Input: part model. Units: mm. Frame: model coordinates. A direction names the side the tool comes from. Coordinates: 2 decimals unless noted, no trailing zeros. Order: outer loops, then holes, each group sorted by start corner. A loop starts at its lowest first (then second) coordinate and runs counter-clockwise, first axis right, second up. Notation, with made-up numbers: M 52,31.5 L 68,31.5 A22 cw 68,40.5 Z; hole C 39.5,69.5 d5. An arc over 180 degrees is marked long. One line per item, written item: value.
Autodesk Inventor part; units mm, degrees
ref_plane "YZ Plane" through (0, 0, 0) normal (1, 0, 0) x (0, 1, 0)
ref_plane "XZ Plane" through (0, 0, 0) normal (0, 1, 0) x (-1, 0, 0)
ref_plane "XY Plane" through (0, 0, 0) normal (0, 0, 1) x (1, 0, 0)
sketch "Эскиз1" plane through (0, 0, 0) normal (0, 1, 0) x (-1, 0, 0)
  circle A0 centre (0, 0) radius 9.815
  dimension "d0" = 19.63
extrude "Выдавливание1" add sketch "Эскиз1" along normal blind 1.33
sketch "Эскиз2" plane through (0, 1.33, 0) normal (0, 1, 0) x (1, 0, 0)
  circle A0 centre (0, 0) radius 3.95
  dimension "d3" = 7.9
extrude "Выдавливание2" add sketch "Эскиз2" along normal blind 2.7
sketch "Эскиз3" plane through (0, 4.03, 0) normal (0, 1, 0) x (1, 0, 0)
  circle A0 centre (0, 0) radius 2.845
  dimension "d6" = 5.69
extrude "Выдавливание3" add sketch "Эскиз3" along normal blind 2.45
fillet "Сопряжение1" radius 2.5 1 edges at (-2.845, 6.48, 0)
sketch "Эскиз4" plane through (0, 1.33, 0) normal (0, 1, 0) x (1, 0, 0)
  circle A0 centre (0, 0) radius 9.815
  line L0 (3.05, 9.815) -> (3.05, -9.815)
  line L1 (-3.05, 9.815) -> (-3.05, -9.815)
  point P0 (-3.05, 9.3291)
  point P1 (-3.05, -9.3291)
  point P2 (3.05, -9.3291)
  point P3 (3.05, 9.3291)
extrude "Выдавливание4" add sketch "Эскиз4" along normal blind 2.6 contours L0 A0 L1
(1) Cut plane A-A on y = 2.25. Output: boundary loops of the cut face in (x, z) (3 decimals), plus the area to 3 significant figures.
Data:
outline: M -3.05,-9.329 A9.815 ccw 3.05,-9.329 L 3.05,-2.51 A3.95 ccw 3.05,2.51 L 3.05,9.329 A9.815 ccw -3.05,9.329 L -3.05,2.51 A3.95 ccw -3.05,-2.51 Z
area: 124 mm2
(2) Cut plane B-B on z = -8. Output: boundary loops of the cut face in (x, y).
Data:
outline: M -5.69,0 L 5.69,0 L 5.69,1.33 L 3.05,1.33 L 3.05,3.93 L -3.05,3.93 L -3.05,1.33 L -5.69,1.33 Z
(3) Ray query, line 1 (Y direction, x = -5.75, z = 3.25); line 2 (X direction, y = 2, z = -6.75); line 3 (Y direction, x = 1.5, z = 9). Return the intervals inside material, ascending. Write a range as from..to.
Data:
line 1: y = 0..1.33
line 2: x = -3.05..3.05
line 3: y = 0..3.93
(4) First-contact query: pin 1 (5 mm diameter, centred on x = -4, z = 0.5, fed in from +Y); pin 2 (3 mm diameter, centred on x = 5.5, y = 1, fed in from +Z); pin 3 (5.5 mm diameter, centred on x = 6.5, z = 1, fed in from +Y). Flat tips, straight axial feed; report the tip coordinate or a pass-through.
Data:
pin 1: stops at y = 6.18
pin 2: stops at z = 8.96
pin 3: stops at y = 4.03
(5) Access query for faces 1 (the flat face through (-3.05, 3, -6)), 2 (the flat face through (-3.05, 3, 6)), 3 (the flat face through (3.05, 3, -6)), 4 (the cylindrical face through (3.65, 2.66, -1.51)), 5 (the flat face through (3.05, 3, 6)). Directions: +Z, -Z, +X, -X, +Y, -Y. A direction counts if a zero-diameter tool reaches every point of the face in a straight line with its end or side. Return the directions, or none.
Data:
face 1: -Z, -X, +Y
face 2: +Z, -X, +Y
face 3: -Z, +X, +Y
face 4: +Y
face 5: +Z, +X, +Y
